Input: part model. Units: mm. Frame: model coordinates. Face numbers are marked on the shaded views. A direction names the side the tool comes from. Round coordinates to 2 decimals unless told otherwise and drop trailing zeros. Write each loop counter-clockwise with the first axis right and the second up, starting at its lowest first coordinate (ties: lowest second). Pieces come first, ordered by that corner, then holes. Notation, with made-up numbers: (63, 59) -> (91, 59) arc R29 cw to (91, 91) -> close; hole circle Ø1 at (0.25, -6.5). An arc over 180 degrees is marked (long way). Use CSV: the item, a comma, the result in double quotes.
```python
from build123d import *

# Parameters (mm, degrees)
SKETCH1_W           = 14.5
SKETCH1_H           = 16
BOSS_EXTRUDE1_DEPTH = 9.4
SKETCH4_W           = 16.813940165
SKETCH4_H           = 16
BOSS_EXTRUDE3_DEPTH = 24.26
SHELL1_T            = -1.3


with BuildPart() as part:
    # Sketch1 → Boss-Extrude1 (new body)
    with BuildSketch(Plane.XY):
        with Locations((7.25, 8)):
            Rectangle(SKETCH1_W, SKETCH1_H)
    extrude(amount=BOSS_EXTRUDE1_DEPTH)

    # Sketch4 → Boss-Extrude3 (add)
    with BuildSketch(Plane.XY.offset(9.4)):
        with Locations((7.249467392, 7.986309029)):
            Rectangle(SKETCH4_W, SKETCH4_H)
    extrude(amount=BOSS_EXTRUDE3_DEPTH)

    # Shell1
    shell1_openings = [part.faces().sort_by_distance(p)[0] for p in [
        (7.25, 8, 0),
    ]]
    offset(amount=SHELL1_T, openings=shell1_openings, kind=Kind.INTERSECTION)


solid = part.part
```
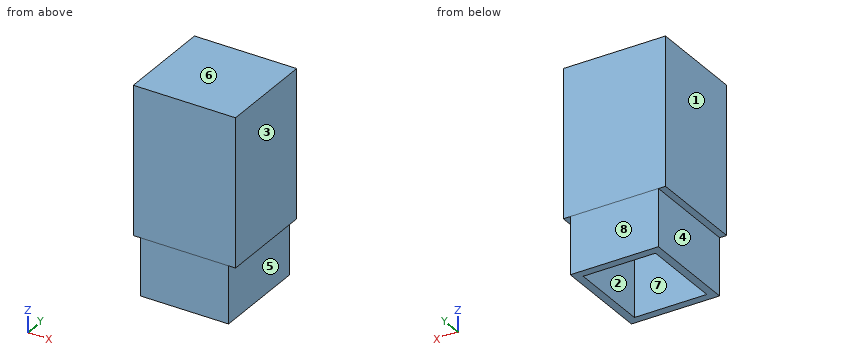
Item 1: Section query C-C on y = 3.75. Return the cut outline in (x, z).
Worked answers:
outline,"(-1.16, 9.4) -> (0, 9.4) -> (0, 0) -> (1.3, 0) -> (1.3, 10.7) -> (0.14, 10.7) -> (0.14, 32.36) -> (14.36, 32.36) -> (14.36, 10.7) -> (13.2, 10.7) -> (13.2, 0) -> (14.5, 0) -> (14.5, 9.4) -> (15.66, 9.4) -> (15.66, 33.66) -> (-1.16, 33.66) -> close"
Item 2: Pull-direction query (Y, two-part tool) for the marked faces 6, 7 and 8; classes: +Y half, -Y half, draft (parallel to the pull), parting line (faces both ways), or undercut.
Worked answers:
face 6,"draft"
face 7,"undercut"
face 8,"+Y half"
Item 3: Section query D-D on z = 11.5. Return the cut outline in (x, y), plus the area to 3 significant figures.
Worked answers:
outline,"(-1.16, -0.01) -> (15.66, -0.01) -> (15.66, 15.99) -> (-1.16, 15.99) -> close; hole (0.14, 1.29) -> (14.36, 1.29) -> (14.36, 14.69) -> (0.14, 14.69) -> close"
area,"78.6 mm²"
Item 4: Section query A-A on z = 7. Return the cut outline in (x, y), plus the area to 3 significant figures.
Worked answers:
outline,"(0, 0) -> (14.5, 0) -> (14.5, 16) -> (0, 16) -> close; hole (1.3, 1.3) -> (13.2, 1.3) -> (13.2, 14.7) -> (1.3, 14.7) -> close"
area,"72.5 mm²"
Item 5: First-contact query: pin 1 Ø4.5 at (x, z) = (6.5, 4) entering from -Y; pin 2 Ø4.5 at (x, z) = (4.5, 22.5) entering from +Y; pin 3 Ø5 at (x, y) = (3, 6) entering from -Z; pin 4 Ø8 at (y, z) = (6.5, 3.5) entering from -X. Flat tips, straight axial feed; report the tip coordinate or a pass-through.
Worked answers:
pin 1,"stops at y = 0"
pin 2,"stops at y = 15.99"
pin 3,"stops at z = 0"
pin 4,"stops at x = 0"
Item 6: Line query: line 1 (X direction, y = 6.5, z = 18.5); line 2 (X direction, y = 4, z = 3); line 3 (Z direction, x = 0.5, y = 12). Output: solid intervals per line, ascending.
Worked answers:
line 1,"x = -1.16 to 0.14, 14.36 to 15.66"
line 2,"x = 0 to 1.3, 13.2 to 14.5"
line 3,"z = 0 to 10.7, 32.36 to 33.66"
Item 7: Set-up query: the marked faces 1, 2, 3, 4 and 5. Return all of +Z, -Z, +X, -X, +Y, -Y with unobstructed straight access to the full face (end or side cutting, diameter ignored); none if empty.
Worked answers:
face 1,"+Z, -Z, -X, +Y, -Y"
face 2,"-Z"
face 3,"+Z, -Z, +X, +Y, -Y"
face 4,"-Z, -X, +Y, -Y"
face 5,"-Z, +X, +Y, -Y"
